Here's the drawing with two shaded views (mm, measured from the low corner). I have some questions. A direction names the side the tool comes from. Coordinates: 2 decimals unless noted, no trailing zeros. Order: outer loops, then holes, each group sorted by start corner. A loop starts at its lowest first (then second) coordinate and runs counter-clockwise, first axis right, second up. Notation, with made-up numbers: (17, -12) - (51, -12) arc R23 ccw to (51, 16) - close; hole circle Ø3 at (59.5, 55.5). An arc over 180 degrees is marked (long way). Answer as a JSON object with one key per item and string values. Group by question number.
(1) Which directions (+Z, -Z, +X, -X, +Y, -Y) give clear straight access to the entire face, cutting with the end or side of a thin tool? Please do the marked faces 1 and 2.
(2) Will these pins go through, and if not, where does the flat tip stop? P1, Ø1.5, axis at x = 27, y = 11.5, coming from the +Z side; P2, Ø6, axis at x = 7.5, y = 27, coming from the +Z side; P3, Ø12, axis at x = 17, z = 64.5, coming from the -Y side.
(3) Imagine slicing it at D-D, the plane z = 56. Write out the boundary of the cut face in (x, y) (1 decimal).
(4) Imagine slicing it at A-A, the plane y = 20. Write out the boundary of the cut face in (x, z).
(5) Please list where these lines run through material, in increasing order: probe 1 along Y at (x, z) = (8.5, 52.5) (1 decimal); probe 2 along X at (y, z) = (14.5, 65) (1 decimal); probe 3 along Z at (x, y) = (14.5, 32) (1 decimal).
(6) Imagine slicing it at C-C, the plane z = 29.5. Write out the boundary of the cut face in (x, y).
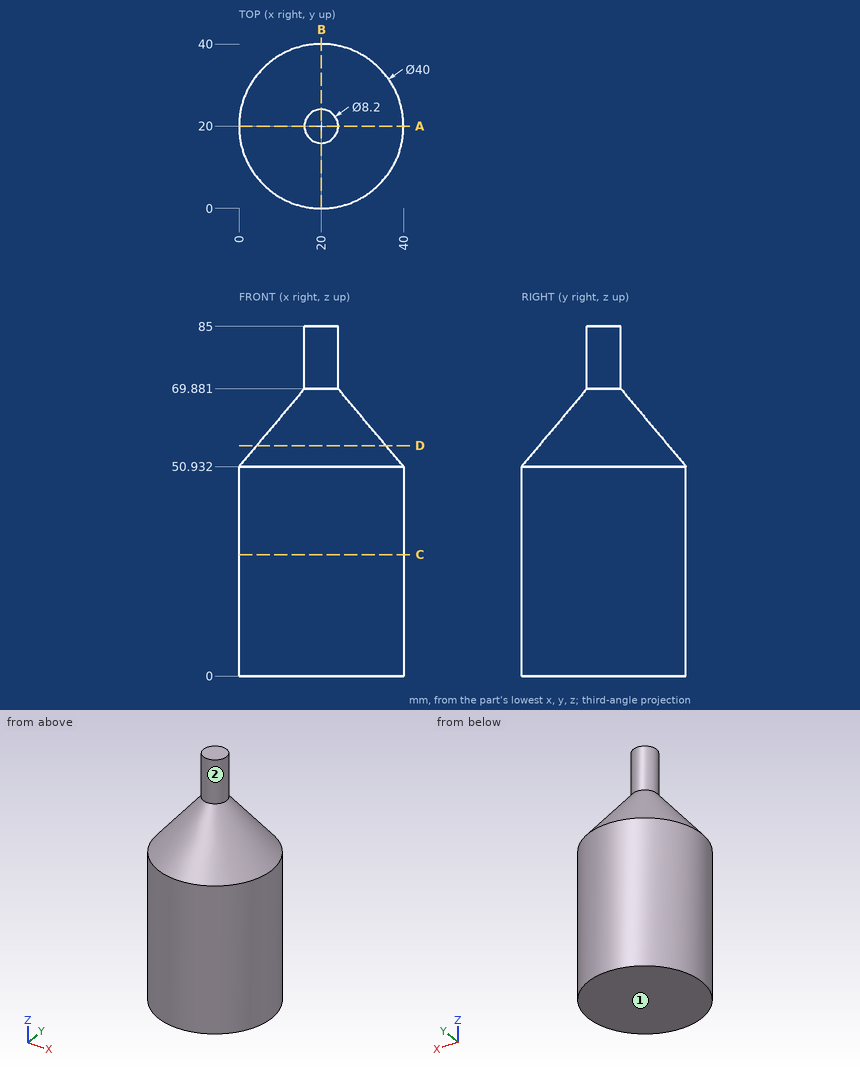
Result set:
{
 "1": {"face 1": "-Z, +X, -X, +Y, -Y", "face 2": "+Z"},
 "2": {"P1": "stops at z = 62.54", "P2": "stops at z = 61.27", "P3": "stops at y = 6.57"},
 "3": {"outline": "circle Ø31.5 at (20, 20)"},
 "4": {"outline": "(0, 0) - (40, 0) - (40, 50.93) - (24.1, 69.88) - (24.1, 85) - (15.9, 85) - (15.9, 69.88) - (0, 50.93) - close"},
 "5": {"probe 1": "y = 5.3 to 34.7", "probe 2": "x = 13.9 to 26.1", "probe 3": "z = 0 to 59"},
 "6": {"outline": "circle Ø40 at (20, 20)"}
}
